Input: part model. Units: mm. Frame: model coordinates. Face numbers are marked on the shaded views. A direction names the side the tool comes from. Round coordinates to 2 decimals unless told otherwise and drop trailing zeros. Loops run counter-clockwise (first coordinate to the right, second up) from the corner with the lowest first, then second, coordinate; pieces in that order, holes last. Notation, with made-up numbers: M -36,13.25 L -6,13.25 A28 cw -6,32.25 Z; hole C 82,16 d8. An arc over 180 degrees is marked long. Return JSON: item names as keys, results as strings. Group by question number.
1) Material intervals for line 1 (Y direction, x = 40, z = -7.5) (3 decimals); line 2 (Z direction, x = 11, y = 3); line 3 (Z direction, x = -34, y = 6.25), sorted ascending. Write a range as from..to.
2) Access query for the marked faces 4 and 5. Directions: +Z, -Z, +X, -X, +Y, -Y. A direction counts if a zero-diameter tool reaches every point of the face in a straight line with its end or side. Return the directions, or none.
3) Contact query for a flat-ended pin moving along its axis: P1, Ø7, axis at x = 0, y = 15.5, coming from the -Z side. Output: stop coordinate, or through.
4) Section B-B (y = 2). Output: boundary loops of the cut face in (x, z), plus the area to 3 significant figures.
5) Section A-A (x = 36.5). Output: boundary loops of the cut face in (y, z) (3 decimals).
6) Section C-C (y = 12.5). Output: boundary loops of the cut face in (x, z), plus the area to 3 significant figures.
7) Mould query, pull axis Y, two halves, no side actions, for the marked faces 1, 2 and 3. Classes: +Y half, -Y half, draft (parallel to the pull), parting line (faces both ways), or undercut.
from build123d import *

# Parameters (mm, degrees)
SKETCH1_W           = 101.6
SKETCH1_H           = 25.4
BOSS_EXTRUDE1_DEPTH = 25.4
SKETCH2_W           = 101.6
SKETCH2_H           = 19.05
CUT_EXTRUDE1_DEPTH  = 22.225
CUT_EXTRUDE2_DEPTH  = 25.4
SKETCH5_R           = 1.524
CUT_EXTRUDE4_DEPTH  = 3.175
CHAMFER1_SIZE       = 0.762
FILLET1_R           = 2.54
FILLET2_R           = 2.54


with BuildPart() as part:
    # Sketch1 → Boss-Extrude1 (new body)
    with BuildSketch(Plane(origin=(0, 0, 0), x_dir=(1, 0, 0), z_dir=(0, 1, 0))):
        with Locations((6.015789474, 0.297076023)):
            Rectangle(SKETCH1_W, SKETCH1_H)
    extrude(amount=BOSS_EXTRUDE1_DEPTH)

    # Sketch2 → Cut-Extrude1 (cut)
    with BuildSketch(Plane(origin=(0, 0, -12.997076023), x_dir=(-1, 0, 0), z_dir=(0, 0, -1))):
        with Locations((-6.015789474, 12.7)):
            Rectangle(SKETCH2_W, SKETCH2_H)
    extrude(amount=-CUT_EXTRUDE1_DEPTH, mode=Mode.SUBTRACT)

    # Sketch4 → Cut-Extrude2 (cut)
    with BuildSketch(Plane(origin=(0, 25.4, 0), x_dir=(1, 0, 0), z_dir=(0, 1, 0))):
        with BuildLine():
            Line((-33.608210526, 0.297076023), (45.639789474, 0.297076023))
            ThreePointArc((45.639789474, 0.297076023), (47.163789474, 1.821076023), (45.639789474, 3.345076023))
            Line((45.639789474, 3.345076023), (-33.608210526, 3.345076023))
            ThreePointArc((-33.608210526, 3.345076023), (-35.132210526, 1.821076023), (-33.608210526, 0.297076023))
        make_face()
    extrude(amount=-CUT_EXTRUDE2_DEPTH, mode=Mode.SUBTRACT)

    # Sketch5 → Cut-Extrude4 (cut)
    with BuildSketch(Plane(origin=(0, 25.4, 0), x_dir=(1, 0, 0), z_dir=(0, 1, 0))):
        with Locations(Location((-19.384210526, 8.425076023, 0), (0, 0, 270))):
            Circle(SKETCH5_R)
        with Locations(Location((-19.384210526, -4.782923977, 0), (0, 0, 270))):
            Circle(SKETCH5_R)
        with Locations(Location((31.415789474, 8.425076023, 0), (0, 0, 270))):
            Circle(SKETCH5_R)
        with Locations(Location((31.415789474, -4.782923977, 0), (0, 0, 270))):
            Circle(SKETCH5_R)
    extrude(amount=-CUT_EXTRUDE4_DEPTH, mode=Mode.SUBTRACT)

    # Chamfer1
    chamfer1_edges = [part.edges().sort_by_distance(p)[0] for p in [
        (-19.384210526, 22.225, -9.949076023),
        (-19.384210526, 22.225, 3.258923977),
        (31.415789474, 22.225, -9.949076023),
        (31.415789474, 22.225, 3.258923977),
    ]]
    chamfer(chamfer1_edges, length=CHAMFER1_SIZE)

    # Fillet1
    fillet1_edges = [part.edges().sort_by_distance(p)[0] for p in [
        (6.015789474, 22.225, 9.227923977),
        (6.015789474, 3.175, 9.227923977),
    ]]
    fillet(fillet1_edges, radius=FILLET1_R)

    # Fillet2
    fillet2_edges = [part.edges().sort_by_distance(p)[0] for p in [
        (-44.784210526, 1.5875, -12.997076023),
        (56.815789474, 1.5875, -12.997076023),
        (-44.784210526, 23.8125, -12.997076023),
        (56.815789474, 23.8125, -12.997076023),
    ]]
    fillet(fillet2_edges, radius=FILLET2_R)


solid = part.part
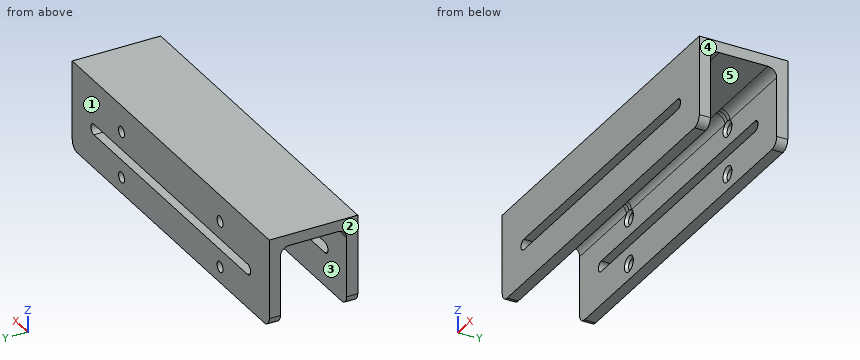
Returned:
{
 "1": {"line 1": "y = 0..3.175, 22.225..25.4", "line 2": "z = -13..-3.35, -0.3..12.4", "line 3": "z = 9.23..12.4"},
 "2": {"face 4": "+Z, -Z, +X, +Y, -Y", "face 5": "-Z, +X, -X"},
 "3": {"P1": "stops at z = 9.23"},
 "4": {"outline": "M -44.78,-10.46 A2.54 ccw -42.24,-13 L 54.28,-13 A2.54 ccw 56.82,-10.46 L 56.82,12.4 L -44.78,12.4 Z; hole M -33.61,-3.35 L 45.64,-3.35 A1.52 ccw 45.64,-0.3 L -33.61,-0.3 A1.52 ccw Z", "area": "2,330 mm^2"},
 "5": {"outline": "M 0,-12.997 L 3.175,-12.997 L 3.175,-3.345 L 0,-3.345 Z; M 0,-0.297 L 3.175,-0.297 L 3.175,6.688 A2.54 cw 5.715,9.228 L 19.685,9.228 A2.54 cw 22.225,6.688 L 22.225,-0.297 L 25.4,-0.297 L 25.4,12.403 L 0,12.403 Z; M 22.225,-12.997 L 25.4,-12.997 L 25.4,-3.345 L 22.225,-3.345 Z"},
 "6": {"outline": "M -44.78,9.23 L 56.82,9.23 L 56.82,12.4 L -44.78,12.4 Z", "area": "323 mm^2"},
 "7": {"face 1": "+Y half", "face 2": "draft", "face 3": "undercut"}
}
